The listing builds one solid part. Answer for the finished solid, in the listing's coordinates (mm). Give positions to 0.01 mm unless a question says otherwise; leave off trailing zeros. Loops run counter-clockwise (first coordinate to the right, second up) from the corner with the lowest first, then second, coordinate; pieces in that order, holes last. Notation, with made-up numbers: (68, -3) - (83, -3) arc R24 ccw to (83, 34) - close; hole circle Ø10 at (24.5, 88.25). An arc over 180 degrees is marked (long way). Write item = value, one per line. Start each with the question number.
1) The part is cut by section A-A on y = 24. Write down the section's boundary in (x, z), plus the area to 3 significant figures.
2) Flat-ended cylindrical pins translate along their axes: P1, Ø6, axis at y = 39, z = 3, coming from the +X side; P2, Ø3, axis at y = 30, z = 0.5, coming from the +X side; P3, Ø1.1, axis at y = 30, z = 0, coming from the +X side; P4, Ø8, axis at x = 26, y = 40.5, coming from the +Z side. Find the tip coordinate at first contact, or state that the pin passes through.
3) The part is cut by section D-D on z = -3.5. Write down the section's boundary in (x, y).
4) The part is cut by section B-B on z = 0.75. Write down the section's boundary in (x, y), plus the area to 3 significant figures.
5) The part is cut by section C-C on x = 53. Write down the section's boundary in (y, z), plus the area to 3 significant figures.
6) Consider probe 1 along Z at (x, y) = (31.5, 10.5); probe 2 along X at (y, z) = (35, 1.5). Determine where each line is inside the solid, lowest interval first.
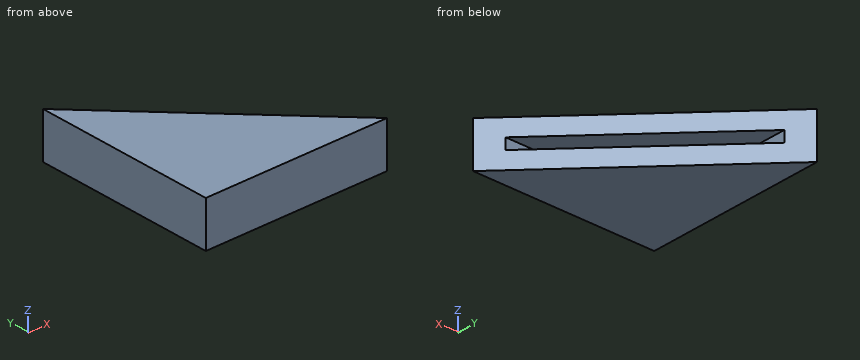
from build123d import *

# Parameters (mm, degrees)
BOSS_EXTRU_1_DEPTH           = 7.5
BOSS_EXTRU_2_DEPTH           = 7.5
ENL_V_MAT_EXTRU_1_DEPTH      = 1.8
ENL_V_MAT_EXTRU_1_DEPTH_BACK = 1.8


with BuildPart() as part:
    # Esquisse1 → Boss.-Extru.1 (new body)
    with BuildSketch(Plane.XY):
        Polygon((0, 0), (0, 60), (60, 0), align=None)
    extrude(amount=BOSS_EXTRU_1_DEPTH)

    # Esquisse4 → Boss.-Extru.2 (add)
    with BuildSketch(Plane(origin=(0, 0, 0), x_dir=(-1, 0, 0), z_dir=(0, 0, -1))):
        Polygon((-60, 0), (0, 0), (0, 60), align=None)
    extrude(amount=BOSS_EXTRU_2_DEPTH)

    # Esquisse5 → Enlèv. mat.-Extru.1 (cut, two sides: drawn at the far end of the back side and taken through both)
    with BuildSketch(Plane.XY.offset(-ENL_V_MAT_EXTRU_1_DEPTH_BACK)):
        Polygon((19.799886626, 5.7), (65.41074544, 5.7), (5.7, 61.280925076), (5.7, 19.989141186), (5.7, 5.7), align=None)
    extrude(amount=ENL_V_MAT_EXTRU_1_DEPTH + ENL_V_MAT_EXTRU_1_DEPTH_BACK, mode=Mode.SUBTRACT)


solid = part.part
Answer below:
q1.outline = (0, -7.5) - (36, -7.5) - (36, -1.8) - (5.7, -1.8) - (5.7, 1.8) - (36, 1.8) - (36, 7.5) - (0, 7.5) - close
q1.area = 431 mm2
q2.P1 = 24
q2.P2 = 30.75
q2.P3 = 5.7
q2.P4 = through
q3.outline = (0, 0) - (60, 0) - (0, 60) - close
q4.outline = (0, 0) - (60, 0) - (54.3, 5.7) - (5.7, 5.7) - (5.7, 54.3) - (0, 60) - close
q4.area = 619 mm2
q5.outline = (0, -7.5) - (7, -7.5) - (7, -1.8) - (5.7, -1.8) - (5.7, 1.8) - (7, 1.8) - (7, 7.5) - (0, 7.5) - close
q5.area = 100 mm2
q6.probe_1 = -7.5 to -1.8, 1.8 to 7.5
q6.probe_2 = 0 to 5.7
